```python
from build123d import *

# Parameters (mm, degrees)
SKETCH_6_W      = 115.2549118
SKETCH_6_H      = 112.856705034
SKETCH_6_R      = 1.75
EXTRUDE_1_DEPTH = 3.6
FILLET_2_R      = 30
FILLET_3_R      = 30


with BuildPart() as part:
    # 草图6 → 凸台-拉伸1 (new body)
    with BuildSketch(Plane(origin=(0, 0, 0), x_dir=(1, 0, 0), z_dir=(0, 1, 0))):
        with Locations((95, 83.571647483)):
            Rectangle(SKETCH_6_W, SKETCH_6_H)
        with BuildLine():
            Line((79.1225441, 41.893294966), (110.8774559, 41.893294966))
            ThreePointArc((110.8774559, 41.893294966), (112.6274559, 40.143294966), (110.8774559, 38.393294966))
            Line((110.8774559, 38.393294966), (79.1225441, 38.393294966))
            ThreePointArc((79.1225441, 38.393294966), (77.3725441, 40.143294966), (79.1225441, 41.893294966))
        make_face(mode=Mode.SUBTRACT)
        with Locations((45.4225441, 32.093294966)):
            Circle(SKETCH_6_R, mode=Mode.SUBTRACT)
        with Locations((69.3225441, 32.093294966)):
            Circle(SKETCH_6_R, mode=Mode.SUBTRACT)
        with Locations((45.4225441, 62.193294966)):
            Circle(SKETCH_6_R, mode=Mode.SUBTRACT)
        with Locations((69.3225441, 62.193294966)):
            Circle(SKETCH_6_R, mode=Mode.SUBTRACT)
        with Locations((120.6774559, 32.093294966)):
            Circle(SKETCH_6_R, mode=Mode.SUBTRACT)
        with Locations((144.5774559, 32.093294966)):
            Circle(SKETCH_6_R, mode=Mode.SUBTRACT)
        with Locations((120.6774559, 62.193294966)):
            Circle(SKETCH_6_R, mode=Mode.SUBTRACT)
        with Locations((144.5774559, 62.193294966)):
            Circle(SKETCH_6_R, mode=Mode.SUBTRACT)
        with BuildLine():
            ThreePointArc((67.429104265, 81.893294966), (65.679104265, 80.143294966), (63.929104265, 81.893294966))
            Line((63.929104265, 81.893294966), (63.929104265, 116.893294966))
            ThreePointArc((63.929104265, 116.893294966), (65.679104265, 118.643294966), (67.429104265, 116.893294966))
            Line((67.429104265, 116.893294966), (67.429104265, 81.893294966))
        make_face(mode=Mode.SUBTRACT)
        with Locations((95, 99.393294966)):
            Circle(SKETCH_6_R, mode=Mode.SUBTRACT)
        with Locations((75.95, 132)):
            Circle(SKETCH_6_R, mode=Mode.SUBTRACT)
        with BuildLine():
            Line((126.070895735, 116.893294966), (126.070895735, 81.893294966))
            ThreePointArc((126.070895735, 81.893294966), (124.320895735, 80.143294966), (122.570895735, 81.893294966))
            Line((122.570895735, 81.893294966), (122.570895735, 116.893294966))
            ThreePointArc((122.570895735, 116.893294966), (124.320895735, 118.643294966), (126.070895735, 116.893294966))
        make_face(mode=Mode.SUBTRACT)
        with Locations((114.05, 132)):
            Circle(SKETCH_6_R, mode=Mode.SUBTRACT)
    extrude(amount=EXTRUDE_1_DEPTH)

    # 圆角2
    fillet_2_edges = [part.edges().sort_by_distance(p)[0] for p in [
        (37.3725441, 1.8, -140),
    ]]
    fillet(fillet_2_edges, radius=FILLET_2_R)

    # 圆角3
    fillet_3_edges = [part.edges().sort_by_distance(p)[0] for p in [
        (152.6274559, 1.8, -140),
    ]]
    fillet(fillet_3_edges, radius=FILLET_3_R)


solid = part.part
```
Read the model definition and answer for the solid it produces. Units are mm, in the model's axes. A direction names the side the tool comes from. Give positions to 0.01 mm unless a question says otherwise; leave off trailing zeros. Write each loop counter-clockwise with the first axis right and the second up, starting at its lowest first coordinate (ties: lowest second). Pieces come first, ordered by that corner, then holes. Notation, with made-up numbers: (-40, -26.5) -> (-4, -26.5) arc R15 cw to (-4, -10.5) -> close; hole circle Ø5 at (-15.75, 32.25). An arc over 180 degrees is marked (long way). Answer as a JSON object with one key per item and string values.
1) Section C-C on y = 2.9 is taken. Count the separate pieces of the cut face and the enclosed holes in it, then the cut area to 3 significant figures.
Findings below:
{"separate pieces": "1", "enclosed holes": "14", "area": "12,100 mm^2"}
2) A flat-ended cylindrical pin translates along its axis: pin 1 Ø2 at (x, z) = (69.32, -62.19) entering from -Y. Find the tip coordinate at first contact, or state that the pin passes through.
Findings below:
{"pin 1": "passes through"}
3) For a pull along X with two mould halves and no side action, classify faces 1 (the flat face through (94, 3.6, -84)), 2 (the flat face through (152.627, 2, -68)), 3 (the cylindrical face through (45.195, 1.775, -63.928)) as pulls with the +X half, pulls with the -X half, needs draft (parallel to the pull), parting line crosses it, or undercut.
Findings below:
{"face 1": "needs draft", "face 2": "pulls with the +X half", "face 3": "undercut"}
4) A tool of negligible diameter and unlimited length cuts with its end or side. For faces 4 (the flat face through (126.071, 2, -100)), 5 (the flat face through (94, 0, -84)), from which of +Z, -Z, +X, -X, +Y, -Y can it reach the whole face along a straight path? Write none if from no direction.
Findings below:
{"face 4": "+Y, -Y", "face 5": "+Z, -Z, +X, -X, -Y"}
5) Straight lines are drawn through the part: probe 1 along Z at (x, y) = (95, 2.25); probe 2 along X at (y, z) = (1.8, -103); probe 3 along Z at (x, y) = (109, 2.75). For each, find the intervals that lie inside material, in ascending order. Write a range as from..to.
Findings below:
{"probe 1": "z = -140..-101.14, -97.64..-41.89, -38.39..-27.14", "probe 2": "x = 37.37..63.93, 67.43..122.57, 126.07..152.63", "probe 3": "z = -140..-41.89, -38.39..-27.14"}
6) Section D-D on z = -132 is taken. Write down the section's boundary in (x, y).
Findings below:
{"outline": "(46.98, 0) -> (74.2, 0) -> (74.2, 3.6) -> (46.98, 3.6) -> close; (77.7, 0) -> (112.3, 0) -> (112.3, 3.6) -> (77.7, 3.6) -> close; (115.8, 0) -> (143.02, 0) -> (143.02, 3.6) -> (115.8, 3.6) -> close"}
7) Section A-A on x = 95 is taken. Write down the section's boundary in (y, z).
Findings below:
{"outline": "(0, -140) -> (3.6, -140) -> (3.6, -101.14) -> (0, -101.14) -> close; (0, -97.64) -> (3.6, -97.64) -> (3.6, -41.89) -> (0, -41.89) -> close; (0, -38.39) -> (3.6, -38.39) -> (3.6, -27.14) -> (0, -27.14) -> close"}
8) Section B-B on x = 75.95 is taken. Write down the section's boundary in (y, z), then the cut area to 3 significant figures.
Findings below:
{"outline": "(0, -140) -> (3.6, -140) -> (3.6, -133.75) -> (0, -133.75) -> close; (0, -130.25) -> (3.6, -130.25) -> (3.6, -27.14) -> (0, -27.14) -> close", "area": "394 mm^2"}
